Could you check a few things on this model? Use its own coordinates, in mm. Coordinates: 2 decimals unless noted, no trailing zeros. Write each loop counter-clockwise with the first axis right and the second up, starting at its lowest first coordinate (ties: lowest second). Pieces come first, ordered by that corner, then holes. Notation, with made-up numbers: (72.25, 68) - (78.25, 68) arc R17 ccw to (78.25, 78) - close; hole circle Ø11 at (77, 75). An arc over 180 degrees is marked (long way). Answer as a JSON object with one key per item and string values. Group by question number.
1) If we section it at D-D (x = 10.75): Write out the boundary of the cut face in (y, z), plus the area to 3 significant figures.
2) If we section it at A-A (y = -0.5): Write out the boundary of the cut face in (x, z).
3) Please list where these lines run through material, in increasing order: line 1 along X through (y, z) = (0, 5); line 2 along X through (y, z) = (-0.55, 25); line 3 along X through (y, z) = (0.3, 4).
4) Will these pins go through, and if not, where does the flat tip stop? pin 1 Ø1.5 at (y, z) = (-0.5, -9.5) entering from -X; pin 2 Ø1.5 at (y, z) = (0.5, -18) entering from +X; pin 3 Ø0.9 at (x, y) = (7.5, 0) entering from -Z.
5) If we section it at C-C (z = -23.5): Write out the boundary of the cut face in (x, y), plus the area to 3 significant figures.
6) If we section it at B-B (x = 0): Write out the boundary of the cut face in (y, z), plus the area to 3 significant figures.
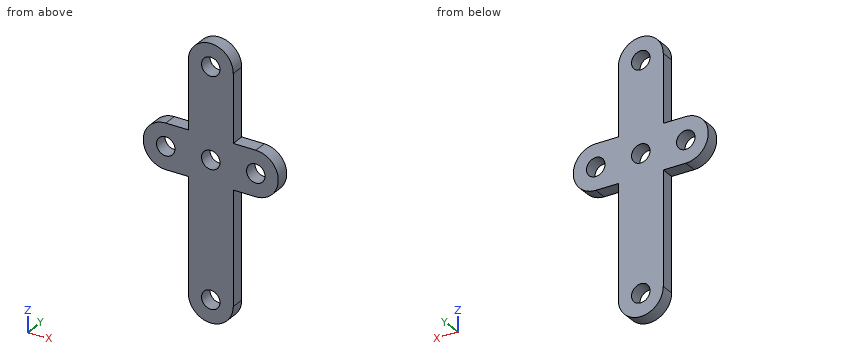
```python
from build123d import *

# Parameters (mm, degrees)
SKETCH1_R           = 2.05
BOSS_EXTRUDE1_DEPTH = 1.5


with BuildPart() as part:
    # Sketch1 → Boss-Extrude1 (new, symmetric)
    with BuildSketch(Plane(origin=(0, 0, 0), x_dir=(1, 0, 0), z_dir=(0, 1, 0))):
        with BuildLine():
            Line((-10, 0), (-5, 0))
            Line((-5, 0), (-5, 25))
            ThreePointArc((-5, 25), (0, 30), (5, 25))
            Line((5, 25), (5, 0))
            Line((5, 0), (10, 0))
            ThreePointArc((10, 0), (15, -5), (10, -10))
            Line((10, -10), (5, -10))
            Line((5, -10), (5, -25))
            ThreePointArc((5, -25), (0, -30), (-5, -25))
            Line((-5, -25), (-5, -10))
            Line((-5, -10), (-10, -10))
            ThreePointArc((-10, -10), (-15, -5), (-10, 0))
        make_face()
        with Locations(Location((10, -5, 0), (0, 0, 270))):
            Circle(SKETCH1_R, mode=Mode.SUBTRACT)
        with Locations(Location((-10, -5, 0), (0, 0, 90))):
            Circle(SKETCH1_R, mode=Mode.SUBTRACT)
        with Locations(Location((0, -5, 0), (0, 0, 270))):
            Circle(SKETCH1_R, mode=Mode.SUBTRACT)
        with Locations(Location((0, 25, 0), (0, 0, 270))):
            Circle(SKETCH1_R, mode=Mode.SUBTRACT)
        with Locations(Location((0, -25, 0), (0, 0, 90))):
            Circle(SKETCH1_R, mode=Mode.SUBTRACT)
    extrude(amount=BOSS_EXTRUDE1_DEPTH, both=True)


solid = part.part
```
Here are the results:
{
 "1": {"outline": "(-1.5, 0.06) - (1.5, 0.06) - (1.5, 3.09) - (-1.5, 3.09) - close; (-1.5, 6.91) - (1.5, 6.91) - (1.5, 9.94) - (-1.5, 9.94) - close", "area": "18.2 mm²"},
 "2": {"outline": "(-10, 0) - (-5, 0) - (-5, -25) arc R5 ccw to (5, -25) - (5, 0) - (10, 0) arc R5 ccw to (10, 10) - (5, 10) - (5, 25) arc R5 ccw to (-5, 25) - (-5, 10) - (-10, 10) arc R5 ccw to start; hole circle Ø4.1 at (-10, 5); hole circle Ø4.1 at (0, -25); hole circle Ø4.1 at (0, 5); hole circle Ø4.1 at (0, 25); hole circle Ø4.1 at (10, 5)"},
 "3": {"line 1": "x = -15 to -12.05, -7.95 to -2.05, 2.05 to 7.95, 12.05 to 15", "line 2": "x = -5 to -2.05, 2.05 to 5", "line 3": "x = -14.9 to -11.79, -8.21 to -1.79, 1.79 to 8.21, 11.79 to 14.9"},
 "4": {"pin 1": "stops at x = -5", "pin 2": "stops at x = 5", "pin 3": "stops at z = 0"},
 "5": {"outline": "(-5, -1.5) - (-1.4, -1.5) - (-1.4, 1.5) - (-5, 1.5) - close; (1.4, -1.5) - (5, -1.5) - (5, 1.5) - (1.4, 1.5) - close", "area": "21.6 mm²"},
 "6": {"outline": "(-1.5, -30) - (1.5, -30) - (1.5, -27.05) - (-1.5, -27.05) - close; (-1.5, -22.95) - (1.5, -22.95) - (1.5, 2.95) - (-1.5, 2.95) - close; (-1.5, 7.05) - (1.5, 7.05) - (1.5, 22.95) - (-1.5, 22.95) - close; (-1.5, 27.05) - (1.5, 27.05) - (1.5, 30) - (-1.5, 30) - close", "area": "143 mm²"}
}
